```python
from build123d import *

# Parameters (mm, degrees)
F0_R     = 5.5
F1_DEPTH = 20
F3_D     = 3.5
F5_DEPTH = 10
F7_DEPTH = 5
F8_R     = 1.99999


# Not quite as in the source:
# - a fillet or chamfer is up to 0.001 mm smaller than in the source, because OpenCascade refuses the exact size


with BuildPart() as f1:
    # F0 (on Top) → F1 (new body)
    with BuildSketch(Plane.XY):
        with BuildLine():
            ThreePointArc((-18, 4), (-14, 0), (-18, -4))
            Line((-18, -4), (-30, -4))
            Line((-30, -4), (-30, -8))
            Line((-30, -8), (-3.8358095935, -14.5012607991))
            ThreePointArc((-3.8358095935, -14.5012607991), (15, 0), (-3.8358095935, 14.5012607991))
            Line((-3.8358095935, 14.5012607991), (-30, 8))
            Line((-30, 8), (-30, 4))
            Line((-30, 4), (-18, 4))
        make_face()
        Circle(F0_R, mode=Mode.SUBTRACT)
    extrude(amount=F1_DEPTH)

    # F3 (through all)
    with Locations(Plane.XY.offset(20)):
        with Locations((8, 0), (0, -8), (-8, 0), (0, 8)):
            Hole(F3_D / 2)

    # F4 (on face) → F5 (cut)
    with BuildSketch(Plane.XY.offset(20)):
        Polygon((11.2331615075, 0), (9.6165807537, 2.8), (6.3834192463, 2.8), (4.7668384925, 0), (6.3834192463, -2.8), (9.6165807537, -2.8), align=None)
        Polygon((-2.8, 9.6165807537), (-2.8, 6.3834192463), (0, 4.7668384925), (2.8, 6.3834192463), (2.8, 9.6165807537), (0, 11.2331615075), align=None)
        Polygon((-9.6165807537, -2.8), (-6.3834192463, -2.8), (-4.7668384925, 0), (-6.3834192463, 2.8), (-9.6165807537, 2.8), (-11.2331615075, 0), align=None)
        Polygon((2.8, -9.6165807537), (2.8, -6.3834192463), (0, -4.7668384925), (-2.8, -6.3834192463), (-2.8, -9.6165807537), (0, -11.2331615075), align=None)
    extrude(amount=-F5_DEPTH, mode=Mode.SUBTRACT)

    # F6 (on face) → F7 (cut)
    with BuildSketch(Plane.XY.offset(20)):
        with BuildLine():
            Line((-6, -13.9635041923), (-3.8358095935, -14.5012607991))
            ThreePointArc((-3.8358095935, -14.5012607991), (15, 0), (-3.8358095935, 14.5012607991))
            Line((-3.8358095935, 14.5012607991), (-6, 13.9635041923))
            Line((-6, 13.9635041923), (-6, 3.5))
            Line((-6, 3.5), (-8, 3.5))
            ThreePointArc((-8, 3.5), (-11.5, 0), (-8, -3.5))
            Line((-8, -3.5), (-6, -3.5))
            Line((-6, -3.5), (-6, -13.9635041923))
        make_face()
    extrude(amount=-F7_DEPTH, mode=Mode.SUBTRACT)

    # F8 (radius 2 in the source; OpenCascade refuses exactly that, so slightly less here)
    f8_edges = [f1.edges().sort_by_distance(p)[0] for p in [
        (-6, -8.731752, 20),
        (-6, 8.731752, 20),
        (-6, -3.5, 17.5),
        (-6, 3.5, 17.5),
    ]]
    fillet(f8_edges, radius=F8_R)


solid = f1.part
```
Input: part model. Units: mm. Frame: model coordinates. A direction names the side the tool comes from. Round coordinates to 2 decimals unless told otherwise and drop trailing zeros. Loops run counter-clockwise (first coordinate to the right, second up) from the corner with the lowest first, then second, coordinate; pieces in that order, holes last. Notation, with made-up numbers: (40.25, 36) - (62.25, 36) arc R9 ccw to (62.25, 53) - close; hole circle Ø7 at (4, -33.5). An arc over 180 degrees is marked (long way). One line per item, written item: value. Start each with the question number.
(1) Section A-A, the plane z = 7. Return loops of the section in (x, y).
(2) Ray query, line 1 (Y direction, x = 0, z = 2); line 2 (X direction, y = -0.5, z = 8.75); line 3 (Y direction, x = -8, z = 7.75). Return the intervals inside material, ascending. Write a range as [from, to].
(3) Contact query for flat-ended pins moving along their axis: P1, Ø1.5, axis at y = -10.5, z = 16, coming from the +X side; P2, Ø1, axis at x = -8, z = 13.5, coming from the -Y side; P3, Ø4.5, axis at x = 0, y = -8, coming from the +Z side; P4, Ø2, axis at x = -8, y = 0, coming from the +Z side. Output: stop coordinate, or through.
(4) Section D-D, the plane y = -10.5. Return loops of the section in (x, z).
(5) Draft query along X for faces 1 (the flat face through (-6, -10, 17)), 2 (the flat face through (-5.895, -1.954, 12.535)), 3 (the cylindrical face through (5.08, -2.11, 7.4)), 4 (the cylindrical face through (15, 0, 7)). Return one class per face: +X half, -X half, draft (parallel to the pull), parting line (faces both ways), or undercut.
(6) Access query for faces 5 (the flat face through (-24, 4, 10)), 6 (the flat face through (-1.42, -10.414, 12.535)), 7 (the cylindrical face through (-6.6, 8.66, 19.43)). Directions: +Z, -Z, +X, -X, +Y, -Y. A direction counts if a zero-diameter tool reaches every point of the face in a straight line with its end or side. Return the directions, or none.
(7) Section B-B, the plane x = -20. Return loops of the section in (y, z), plus the area to 3 significant figures.
Results below:
1. outline: (-30, -8) - (-3.84, -14.5) arc R15 ccw (long way) to (-3.84, 14.5) - (-30, 8) - (-30, 4) - (-18, 4) arc R4 cw to (-18, -4) - (-30, -4) - close; hole circle Ø3.5 at (-8, 0); hole circle Ø11 at (0, 0); hole circle Ø3.5 at (0, -8); hole circle Ø3.5 at (0, 8); hole circle Ø3.5 at (8, 0)
2. line 1: [-15, -9.75], [-6.25, -5.5], [5.5, 6.25], [9.75, 15]
2. line 2: [-14.03, -9.68], [-6.32, -5.48], [5.48, 6.32], [9.68, 14.99]
2. line 3: [-13.47, -1.75], [1.75, 13.47]
3. P1: x = -6
3. P2: y = -13.59
3. P3: z = 10
3. P4: through
4. outline: (-19.94, 0) - (10.71, 0) - (10.71, 15) - (1.27, 15) - (1.27, 10) - (-1.27, 10) - (-1.27, 15) - (-6, 15) - (-6, 18) arc R2 ccw to (-8, 20) - (-19.94, 20) - close
5. face 1: +X half
5. face 2: undercut
5. face 3: undercut
5. face 4: parting line
6. face 5: +Z, -Z, -X
6. face 6: +Z
6. face 7: +Z, +X, +Y, -Y
7. outline: (-10.48, 0) - (-4, 0) - (-4, 20) - (-10.48, 20) - close; (4, 0) - (10.48, 0) - (10.48, 20) - (4, 20) - close
7. area: 259 mm^2
